Read the model definition and answer for the solid it produces. Units are mm, in the model's axes. Give positions to 0.01 mm unless a question says otherwise; leave off trailing zeros. Order: outer loops, then holes, each group sorted by start corner. A loop starts at its lowest first (then second) coordinate and runs counter-clockwise, first axis right, second up. Notation, with made-up numbers: M 2,-7 L 14,-7 A16 ccw 14,2 Z; hole C -21,78 d2. An arc over 180 degrees is marked long. One line per item, written item: value.
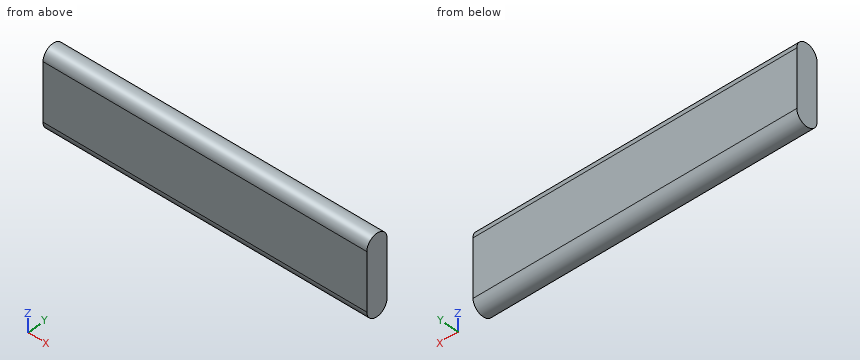
from build123d import *

# Parameters (mm, degrees)
SKETCH_1_W      = 82
SKETCH_1_H      = 20
EXTRUDE_1_DEPTH = 5.5
FILLET_1_RADIUS = 2.75
FILLET_1_LENGTH = 82
FILLET_2_RADIUS = 2.75
FILLET_2_LENGTH = 82


with BuildPart() as part:
    # 草图1 → 凸台-拉伸1 (new body)
    with BuildSketch(Plane(origin=(0, 0, 0), x_dir=(1, 0, 0), z_dir=(0, 1, 0))):
        with Locations((41, -10)):
            Rectangle(SKETCH_1_W, SKETCH_1_H)
    extrude(amount=EXTRUDE_1_DEPTH)

    # 圆角1: full round fillet: the end face becomes a half cylinder, R = half its width
    fillet_1_face = Plane((41, 2.75, 0), x_dir=(1, 0, 0), z_dir=(0, 0, -1))  # on the end face: x along it, z out of the body
    fillet_1_slab = fillet_1_face.offset(-FILLET_1_RADIUS / 2) * Box(FILLET_1_LENGTH, 2 * FILLET_1_RADIUS, FILLET_1_RADIUS, mode=Mode.PRIVATE)  # the body's end, R deep
    fillet_1_round = Plane((41, 2.75, 2.75), x_dir=(0, 0, -1), z_dir=(1, 0, 0)) * Cylinder(FILLET_1_RADIUS, FILLET_1_LENGTH, mode=Mode.PRIVATE)  # its axis R under the face
    add(fillet_1_slab - fillet_1_round, mode=Mode.SUBTRACT)

    # 圆角2: full round fillet: the end face becomes a half cylinder, R = half its width
    fillet_2_face = Plane((41, 2.75, 20), x_dir=(1, 0, 0), z_dir=(0, 0, 1))  # on the end face: x along it, z out of the body
    fillet_2_slab = fillet_2_face.offset(-FILLET_2_RADIUS / 2) * Box(FILLET_2_LENGTH, 2 * FILLET_2_RADIUS, FILLET_2_RADIUS, mode=Mode.PRIVATE)  # the body's end, R deep
    fillet_2_round = Plane((41, 2.75, 17.25), x_dir=(0, 0, 1), z_dir=(1, 0, 0)) * Cylinder(FILLET_2_RADIUS, FILLET_2_LENGTH, mode=Mode.PRIVATE)  # its axis R under the face
    add(fillet_2_slab - fillet_2_round, mode=Mode.SUBTRACT)


solid = part.part
1) Find section B-B, the plane y = 4.7. Write down the section's boundary in (x, z).
Reported:
outline: M 0,0.81 L 82,0.81 L 82,19.19 L 0,19.19 Z
2) Find section A-A, the plane x = 48.5. Write down the section's boundary in (y, z), plus the area to 3 significant figures.
Reported:
outline: M 0,2.75 A2.75 ccw 5.5,2.75 L 5.5,17.25 A2.75 ccw 0,17.25 Z
area: 104 mm^2
3) Consider probe 1 along Z at (x, y) = (58, 2.9); probe 2 along Z at (x, y) = (66, 4.4); probe 3 along Y at (x, z) = (54, 1.5). Determine where each line is inside the solid, lowest interval first.
Reported:
probe 1: z = 0 to 20
probe 2: z = 0.55 to 19.45
probe 3: y = 0.3 to 5.2
